Work out the finished part from the listing and answer in its coordinate system (mm). A direction names the side the tool comes from. Coordinates: 2 decimals unless noted, no trailing zeros. Loops run counter-clockwise (first coordinate to the right, second up) from the corner with the lowest first, then second, coordinate; pieces in that order, holes last. Notation, with made-up numbers: M 71.5,51 L 116.5,51 A17 cw 116.5,56 Z; hole C -21,82 d3. An arc over 180 degrees is marked long. Write each question's results on one line, items separated by ' | '.
```python
from build123d import *
from build123d.topology import SkipClean

# Parameters (mm, degrees)
BOSS_EXTRUDE1_DEPTH      = 20.574
BOSS_EXTRUDE1_DEPTH_BACK = 20.574
SKETCH1_W                = 34.798
SKETCH1_H                = 45.974
SKETCH1_R                = 10.414
HOLE1_D                  = 3.96748
HOLE1_DEPTH              = 11.5824
HOLE1_CSINK_D            = 4.826
HOLE1_CSINK_ANGLE        = 90
HOLE1_TIP                = 1.145312823
HOLE2_D                  = 3.96748
HOLE2_DEPTH              = 11.5824
HOLE2_CSINK_D            = 4.826
HOLE2_CSINK_ANGLE        = 90
HOLE2_TIP                = 1.145312823
HOLE3_D                  = 9.525
HOLE3_CBORE_D            = 22.2758
HOLE3_CBORE_DEPTH        = 24.638
HOLE4_D                  = 3.7592
HOLE4_DEPTH              = 7.5184
LPATTERN2_START          = 13.0556
LPATTERN2_OUTLINE_R      = 1.8796
LPATTERN2_DEPTH          = 7.5184
HOLE5_D                  = 3.7592
HOLE5_DEPTH              = 7.5184
LPATTERN4_START          = -20.574
LPATTERN4_OUTLINE_R      = 1.8796
LPATTERN4_DEPTH          = 7.5184


# Read off the part's stored shape, not the designer's step: LPattern2, LPattern4
with BuildPart() as part:
    # Sketch1 → Boss-Extrude1 (new, two sides: drawn at the far end of the back side and taken through both)
    with BuildSketch(Plane(origin=(0, 0, 0), x_dir=(0, 0, -1), z_dir=(1, 0, 0)).offset(-BOSS_EXTRUDE1_DEPTH_BACK)):
        with Locations((0, 22.987)):
            Rectangle(SKETCH1_W, SKETCH1_H)
        with Locations((0, 18.542)):
            Circle(SKETCH1_R, mode=Mode.SUBTRACT)
    extrude(amount=BOSS_EXTRUDE1_DEPTH + BOSS_EXTRUDE1_DEPTH_BACK)

    # Sketch2 → Cut-Revolve1 (revolve, cut)
    with BuildSketch(Plane(origin=(15.875, 0, 0), x_dir=(0, 0, -1), z_dir=(1, 0, 0)), mode=Mode.PRIVATE) as cut_revolve1_sk:
        Polygon((-17.399, 31.75), (-17.399, 35.9029), (-12.319, 35.9029), (-12.319, 34.3296875), (12.319, 34.3296875), (12.319, 35.9029), (17.399, 35.9029), (17.399, 31.75), align=None)
    revolve(cut_revolve1_sk.sketch.rotate(Axis((15.875, 31.75, -17.399), (0, 0, 1)), 270), axis=Axis((15.875, 31.75, -17.399), (0, 0, 1)), mode=Mode.SUBTRACT)

    # Sketch3 → Cut-Revolve2 (revolve, cut)
    with BuildSketch(Plane(origin=(-15.875, 0, 0), x_dir=(0, 0, -1), z_dir=(1, 0, 0)), mode=Mode.PRIVATE) as cut_revolve2_sk:
        Polygon((-17.399, 31.75), (-17.399, 35.9029), (-12.319, 35.9029), (-12.319, 34.3296875), (12.319, 34.3296875), (12.319, 35.9029), (17.399, 35.9029), (17.399, 31.75), align=None)
    revolve(cut_revolve2_sk.sketch.rotate(Axis((-15.875, 31.75, -17.399), (0, 0, 1)), 270), axis=Axis((-15.875, 31.75, -17.399), (0, 0, 1)), mode=Mode.SUBTRACT)

    # Hole1
    with Locations(Plane(origin=(0, 0, 0), x_dir=(-1, 0, 0), z_dir=(0, -1, 0))):
        with Locations((0, -12.7)):
            CounterSinkHole(HOLE1_D / 2, HOLE1_CSINK_D / 2, depth=HOLE1_DEPTH, counter_sink_angle=HOLE1_CSINK_ANGLE)
            with Locations((0, 0, -(HOLE1_DEPTH + HOLE1_TIP / 2))):  # 120° drill point
                Cone(0, HOLE1_D / 2, HOLE1_TIP, mode=Mode.SUBTRACT)

    # Hole2
    with Locations(Plane(origin=(0, 0, 0), x_dir=(-1, 0, 0), z_dir=(0, -1, 0))):
        with Locations((0, 12.7)):
            CounterSinkHole(HOLE2_D / 2, HOLE2_CSINK_D / 2, depth=HOLE2_DEPTH, counter_sink_angle=HOLE2_CSINK_ANGLE)
            with Locations((0, 0, -(HOLE2_DEPTH + HOLE2_TIP / 2))):  # 120° drill point
                Cone(0, HOLE2_D / 2, HOLE2_TIP, mode=Mode.SUBTRACT)

    # Hole3 (through all)
    with Locations(Plane.XY.offset(17.399)):
        with Locations((0, 31.75)):
            CounterBoreHole(HOLE3_D / 2, HOLE3_CBORE_D / 2, HOLE3_CBORE_DEPTH)

    # Sketch10 → Revolve1 (revolve)
    with SkipClean():  # the faces are left unmerged after this step: merging them gives an invalid solid
        with BuildSketch(Plane(origin=(0, 0, 0), x_dir=(0, 0, -1), z_dir=(1, 0, 0)), mode=Mode.PRIVATE) as revolve1_sk:
            Polygon((-18.923, 42.3545), (-18.923, 36.5125), (7.239, 36.5125), (7.239, 42.8625), (-18.415, 42.8625), align=None)
        revolve(revolve1_sk.sketch.rotate(Axis((0, 31.75, -7.239), (0, 0, 1)), 270), axis=Axis((0, 31.75, -7.239), (0, 0, 1)))
    add(part.part.scale(1), mode=Mode.REPLACE)  # the faces are merged on a copy

    # Hole4
    with Locations(Plane(origin=(20.574, 0, 0), x_dir=(0, 0, -1), z_dir=(1, 0, 0))):
        with Locations((13.108504848, 25.511915663)):
            Hole(HOLE4_D / 2, depth=HOLE4_DEPTH)

    # LPattern2 outline → LPattern2 (cut)
    with BuildSketch(Plane.YZ.offset(LPATTERN2_START)):
        with Locations((3.6957, 0)):
            Circle(LPATTERN2_OUTLINE_R)
        with Locations((25.511915663, 13.108504848)):
            Circle(LPATTERN2_OUTLINE_R)
    extrude(amount=LPATTERN2_DEPTH, mode=Mode.SUBTRACT)

    # Hole5
    with Locations(Plane.ZY.offset(20.574)):
        with Locations((-13.108504848, 25.511915663)):
            Hole(HOLE5_D / 2, depth=HOLE5_DEPTH)

    # LPattern4 outline → LPattern4 (cut)
    with BuildSketch(Plane.YZ.offset(LPATTERN4_START)):
        with Locations((3.6957, 0)):
            Circle(LPATTERN4_OUTLINE_R)
        with Locations((25.511915663, 13.108504848)):
            Circle(LPATTERN4_OUTLINE_R)
    extrude(amount=LPATTERN4_DEPTH, mode=Mode.SUBTRACT)


solid = part.part
```
1) Straight lines are drawn through the part: probe 1 along Z at (x, y) = (0, 5); probe 2 along Y at (x, z) = (17.5, 7); probe 3 along Y at (x, z) = (4, -8). For each, find the intervals that lie inside material, in ascending order. Write a range as [from, to].
Check result:
probe 1: [-17.4, -14.68], [-10.72, 10.72], [14.68, 17.4] | probe 2: [0, 10.83], [26.25, 29.75], [33.75, 45.97] | probe 3: [0, 11.87], [25.21, 29.17], [34.33, 45.97]
2) Find section A-A, the plane z = 16. Give the number of separate pieces and of enclosed holes in the cut face, and give its area (3 significant figures).
Check result:
separate pieces: 2 | enclosed holes: 4 | area: 1,710 mm^2
3) Find section D-D, the plane y = 15.5. Give the vertices of the cut face in (x, z).
Check result:
outline: M -20.57,-17.4 L 20.57,-17.4 L 20.57,-9.96 L -20.57,-9.96 Z; M -20.57,9.96 L 20.57,9.96 L 20.57,17.4 L -20.57,17.4 Z
4) Given pin 1 Ø1.9 at (y, z) = (3, -0.5) entering from +X; pin 2 Ø13.5 at (x, y) = (15.875, 31.75) entering from -Z; pin 3 Ø1.1 at (y, z) = (25.5, 12) entering from -X; pin 4 Ø5.5 at (x, y) = (0, 31.75) entering from -Z (3 decimals), each flat-ended and moving along its own axis, determine where each tip first touches the part or whether it passes through.
Check result:
pin 1: x = 13.06 | pin 2: z = -17.4 | pin 3: x = -13.06 | pin 4: through
5) Which of the six approach directions +Z, -Z, +X, -X, +Y, -Y give full straight-line access (tool end or side, diameter ignored) to faces 5 (the face through (-0.43, 6.084, -10.763)), 6 (the face through (16.76, 24.13, 14.38)), 7 (the face through (-12.04, 30.16, 14.82))?
Check result:
face 5: -Y | face 6: +X | face 7: +Z
6) Find section B-B, the plane x = 14.5. Give the vertices of the cut face in (y, z), and give its area (3 significant figures).
Check result:
outline: M 0,-17.4 L 27.83,-17.4 L 27.83,-12.32 L 29.57,-12.32 L 29.57,12.32 L 27.83,12.32 L 27.83,17.4 L 0,17.4 Z; M 33.93,-12.32 L 35.67,-12.32 L 35.67,-17.4 L 45.97,-17.4 L 45.97,17.4 L 35.67,17.4 L 35.67,12.32 L 33.93,12.32 Z; hole C 3.7,0 d3.76; hole C 18.54,0 d20.83; hole C 25.51,-13.11 d3.76; hole C 25.51,13.11 d3.76 | area: 1,040 mm^2
7) For a pull along Z with two mould halves and no side action, classify faces 1 (the face through (0, 18, 17.399)), 2 (the face through (0.04, 12.53, -13.04)), 3 (the face through (-13.056, 4, 0)), 4 (the face through (0, 23, -17.399)) as released by +Z, released by -Z, zero draft, split by the parting line, or undercut.
Check result:
face 1: released by +Z | face 2: undercut | face 3: undercut | face 4: released by -Z
